Model file for the job. Use its own axes, mm. A direction names the side the tool comes from. Coordinates: 2 decimals unless noted, no trailing zeros. Write each loop counter-clockwise with the first axis right and the second up, starting at its lowest first coordinate (ties: lowest second). Pieces come first, ordered by that corner, then holes. Notation, with made-up numbers: (43, 86) -> (64, 86) arc R32 ccw to (64, 118) -> close; hole circle Ø9 at (81.25, 1). An arc over 180 degrees is marked (long way). Write item = value, one per line. Start each with the question number.
from build123d import *

# Parameters (mm, degrees)
F0_W           = 304.8
F0_H           = 76.3
F1_DEPTH       = 3
F2_DEPTH       = 76.2
F3_T1_DEPTH    = 173.7
F4_R           = 19.5
F5_T1_DEPTH    = 479.4867573526
F6_R           = 20.0387150069
F8_R           = 12.7
F9_DEPTH       = 10
F9_DEPTH_BACK  = 86
F10_R          = 12.7
F11_DEPTH      = 10
F11_DEPTH_BACK = 86


# Not quite as in the source:
# - a fillet or chamfer that OpenCascade refuses, or shapes differently, is made with other operations: its cross-section is extruded or revolved along the edge and cut away or added


with BuildPart() as f1:
    # F0 (on Right) → F1 (new body)
    with BuildSketch(Plane.YZ):
        with Locations((152.4, 38.15)):
            Rectangle(F0_W, F0_H)
    extrude(amount=F1_DEPTH)

    # F0 (on Right) → F2 (join)
    with BuildSketch(Plane.YZ):
        with Locations((152.4, 38.15)):
            Rectangle(F0_W, F0_H)
    extrude(amount=F2_DEPTH)

    # F3: fillet of radius 19.5 on 1 edges, made by hand

    # F3_s2 → F3_t1 (cut)
    with BuildSketch(Plane.YZ.offset(-48.75)):
        with BuildLine():
            add(Edge.make_bspline(
                [(0, 19.5), (0, 0), (19.5, 0)],
                knots=[0, 0, 0, 1, 1, 1], degree=2, weights=[1, 1, 1]))
            Line((19.5, 0), (0, 0))
            Line((0, 0), (0, 19.5))
        make_face()
    extrude(amount=F3_T1_DEPTH, mode=Mode.SUBTRACT)

    # F4
    f4_edges = [f1.edges().sort_by_distance(p)[0] for p in [
        (38.1, 304.8, 76.3),
    ]]
    fillet(f4_edges, radius=F4_R)

    # F5: chamfer of 45 x 77.9422863406 on 1 edges, made by hand

    # F5_s2 → F5_t1 (cut)
    with BuildSketch(Plane.YZ.offset(-201.6433786763)):
        Polygon((77.9422863406, 76.3), (0, 31.3), (0, 76.3), align=None)
    extrude(amount=F5_T1_DEPTH, mode=Mode.SUBTRACT)

    # F6
    f6_edges = [f1.edges().sort_by_distance(p)[0] for p in [
        (38.1, 0, 31.3),
    ]]
    fillet(f6_edges, radius=F6_R)

    # F8 (on offset) → F9 (join, two sides)
    with BuildSketch(Plane.YZ.offset(76.2)) as f9_sk:
        with Locations((19.4881175538, 19.05)):
            Circle(F8_R)
    extrude(amount=F9_DEPTH)
    extrude(f9_sk.sketch, amount=-F9_DEPTH_BACK)

    # F10 (on offset) → F11 (join, two sides)
    with BuildSketch(Plane.YZ.offset(76.2)) as f11_sk:
        with Locations((285.75, 57.25)):
            Circle(F10_R)
    extrude(amount=F11_DEPTH)
    extrude(f11_sk.sketch, amount=-F11_DEPTH_BACK)


solid = f1.part
(1) Saw through at B-B (y = 260). Give the cut face in (x, z).
(2) 3-axis set-ups, long thin cutter, end or side, ignore diameter. For faces 1 (the face through (38, 304.8, 28)), 2 (the face through (81.13, 297.864, 61.065)), 3 (the face through (-4.83, 16.74, 6.65)): which of +Z, -Z, +X, -X, +Y, -Y reach the whole face in a straight line?
(3) Drill centre lines: line 1 along X through (y, z) = (138.5, 32.5); line 2 along Y through (x, z) = (39, 18); line 3 along Y through (x, z) = (31.5, 49). Where is each one in solid material? Low to high.
(4) Drop flat-ended pins along their axis: pin 1 Ø5 at (y, z) = (266.5, 52) entering from -X; pin 2 Ø23 at (y, z) = (135, 29.5) entering from +X; pin 3 Ø4 at (x, z) = (36, 51) entering from -Y. Give the stop position or say it passes through.
(5) Saw through at C-C (y = 71.5). Give the cut face in (x, z).
(6) Saw through at A-A (z = 50.5). Give the cut face in (x, y).
Returned:
q1.outline = (0, 0) -> (76.2, 0) -> (76.2, 76.3) -> (0, 76.3) -> close
q2.face_1 = +Z, -Z, +X, -X, +Y
q2.face_2 = +X
q2.face_3 = -X
q3.line_1 = 0 to 76.2
q3.line_2 = 0.03 to 304.8
q3.line_3 = 30.66 to 304.8
q4.pin_1 = 0
q4.pin_2 = 76.2
q4.pin_3 = 30.66
q5.outline = (0, 0) -> (76.2, 0) -> (76.2, 72.58) -> (0, 72.58) -> close
q6.outline = (-9.8, 274.99) -> (0, 274.99) -> (0, 33.26) -> (76.2, 33.26) -> (76.2, 274.99) -> (86.2, 274.99) -> (86.2, 296.51) -> (76.2, 296.51) -> (76.2, 304.8) -> (0, 304.8) -> (0, 296.51) -> (-9.8, 296.51) -> close
